Geometry: final body of the model. Coordinates: model frame, mm. A direction names the side the tool comes from. Coordinates: 2 decimals unless noted, no trailing zeros. Loops run counter-clockwise (first coordinate to the right, second up) from the corner with the lowest first, then second, coordinate; pieces in that order, holes last. Notation, with made-up numbers: (36.5, 12.25) - (77.5, 12.25) arc R10 cw to (77.5, 28.25) - close; hole circle Ø2 at (59, 25.25). An arc over 180 degrees is marked (long way). Return JSON: item names as keys, results as strings.
from build123d import *

# Parameters (mm, degrees)
F1_DEPTH = 35
F2_R     = 15
F3_DEPTH = 10
F4_DEPTH = 32
F5_R     = 4


with BuildPart() as f1:
    # F0 (on Front) → F1 (new body)
    with BuildSketch(Plane.XZ):
        Polygon((60, 0), (0, 0), (0, -35), (15, -45), (45, -45), (60, -35), align=None)
    extrude(amount=F1_DEPTH)

    # F2 (on face) → F3 (cut)
    with BuildSketch(Plane.XZ.offset(35)):
        Polygon((58, -2), (2, -2), (2, -33.5), (15.5, -43), (30, -43), (44.5, -43), (58, -33.5), align=None)
        with Locations((30, -26.5)):
            Circle(F2_R, mode=Mode.SUBTRACT)
    extrude(amount=-F3_DEPTH, mode=Mode.SUBTRACT)

    # F4 (cut): faces of the model
    f4_faces = [f1.faces().sort_by_distance(p)[0] for p in [
        (30, -35, -26.5),
        (30, -35, -26.5),
    ]]
    extrude(f4_faces, amount=-F4_DEPTH, mode=Mode.SUBTRACT)

    # F5
    f5_edges = [f1.edges().sort_by_distance(p)[0] for p in [
        (60, -17.5, 0),
        (60, -17.5, -35),
        (0, -17.5, 0),
        (45, -17.5, -45),
        (15, -17.5, -45),
        (0, -17.5, -35),
        (2, -30, -33.5),
        (44.5, -30, -43),
        (15.5, -30, -43),
        (58, -30, -33.5),
        (58, -30, -2),
        (2, -30, -2),
    ]]
    fillet(f5_edges, radius=F5_R)


solid = f1.part
Item 1: Ray query, probe 1 along X at (y, z) = (-27, -26); probe 2 along Z at (x, y) = (30, -11); probe 3 along X at (y, z) = (-13, -27). Return the intervals inside material, ascending. Write a range as from..to.
Worked out:
{"probe 1": "0..2, 58..60", "probe 2": "-45..-41.5, -11.5..0", "probe 3": "0..15.01, 44.99..60"}
Item 2: Section query B-B, the plane x = 30. Return loops of the section in (y, z), and give its area (3 significant figures).
Worked out:
{"outline": "(-35, -45) - (0, -45) - (0, 0) - (-35, 0) - (-35, -2) - (-25, -2) - (-25, -11.5) - (-3, -11.5) - (-3, -41.5) - (-25, -41.5) - (-25, -43) - (-35, -43) - close", "area": "505 mm^2"}
Item 3: Mould query, pull axis X, two halves, no side actions, for faces 1 (the face through (30, 0, -22)), 2 (the face through (58.797, -17.745, -1.141)), 3 (the face through (44.42, -29.93, -42.82)). Classes: +X half, -X half, draft (parallel to the pull), parting line (faces both ways), or undercut.
Worked out:
{"face 1": "draft", "face 2": "+X half", "face 3": "undercut"}
Item 4: Section query C-C, the plane z = -26.5. Return loops of the section in (x, y), and give its area (3 significant figures).
Worked out:
{"outline": "(0, -35) - (2, -35) - (2, -25) - (15, -25) - (15, -3) - (45, -3) - (45, -25) - (58, -25) - (58, -35) - (60, -35) - (60, 0) - (0, 0) - close", "area": "880 mm^2"}
Item 5: Section query D-D, the plane y = -17. Return loops of the section in (x, z), and give its area (3 significant figures).
Worked out:
{"outline": "(0, -32.86) arc R4 ccw to (1.78, -36.19) - (13.99, -44.33) arc R4 ccw to (16.21, -45) - (43.79, -45) arc R4 ccw to (46.01, -44.33) - (58.22, -36.19) arc R4 ccw to (60, -32.86) - (60, -4) arc R4 ccw to (56, 0) - (4, 0) arc R4 ccw to (0, -4) - close; hole circle Ø30 at (30, -26.5)", "area": "1,830 mm^2"}
Item 6: Section query A-A, the plane y = -29. Return loops of the section in (x, z), and give its area (3 significant figures).
Worked out:
{"outline": "(0, -32.86) arc R4 ccw to (1.78, -36.19) - (13.99, -44.33) arc R4 ccw to (16.21, -45) - (43.79, -45) arc R4 ccw to (46.01, -44.33) - (58.22, -36.19) arc R4 ccw to (60, -32.86) - (60, -4) arc R4 ccw to (56, 0) - (4, 0) arc R4 ccw to (0, -4) - close; hole (2, -31.42) arc R4 ccw to (3.7, -34.69) - (14.46, -42.27) arc R4 ccw to (16.77, -43) - (43.23, -43) arc R4 ccw to (45.54, -42.27) - (56.3, -34.69) arc R4 ccw to (58, -31.42) - (58, -6) arc R4 ccw to (54, -2) - (6, -2) arc R4 ccw to (2, -6) - close", "area": "382 mm^2"}
Item 7: Reachability of faces 4 (the face through (3.203, -29.93, -3.141)), 5 (the face through (44.964, -17.745, -44.824)) from +Z, -Z, +X, -X, +Y, -Y: full face, straight path, thin tool, end or side. Return the list, or none.
Worked out:
{"face 4": "-Y", "face 5": "-Z, +X, +Y, -Y"}
Item 8: First-contact query: pin 1 Ø12 at (x, z) = (53.5, -17.5) entering from -Y; pin 2 Ø12.5 at (x, z) = (33.5, -16.5) entering from -Y; pin 3 Ø2 at (x, y) = (46, -5.5) entering from -Z. Flat tips, straight axial feed; report the tip coordinate or a pass-through.
Worked out:
{"pin 1": "y = -35", "pin 2": "y = -25", "pin 3": "z = -44.81"}
